Here's how the part is built. I have some questions about the finished solid (model axes, mm). Face numbers are marked on the shaded views. A direction names the side the tool comes from. Give positions to 0.01 mm unless a question says otherwise; leave off trailing zeros. Loops run counter-clockwise (first coordinate to the right, second up) from the corner with the lowest first, then second, coordinate; pieces in that order, holes last. Notation, with made-up numbers: (52, 26) - (66, 26) arc R29 ccw to (66, 65) - close; hole circle Ø4 at (56, -3.75). An arc over 180 degrees is marked (long way). Use a Markdown table: item, result.
from build123d import *

# Parameters (mm, degrees)
CYLINDER_R        = 1.45
CYLINDER_DEPTH    = 20
ARRAY_Y_COUNT     = 2
ARRAY_Y_PITCH     = 9
BOX002_W          = 5
BOX002_H          = 14.5
BOX002_DEPTH      = 2
BOX003_W          = 2
BOX003_H          = 14.5
BOX003_DEPTH      = 2
CYLINDER001_R     = 1.8
CYLINDER001_DEPTH = 10
ARRAY002_Y_COUNT  = 2
ARRAY002_Y_PITCH  = 30
BOX004_W          = 9.6
BOX004_H          = 40
BOX004_DEPTH      = 2
FILLET_R          = 4
BOX001_W          = 16
BOX001_H          = 14.5
BOX001_DEPTH      = 3.5
BOX_W             = 17
BOX_H             = 16.5
BOX_DEPTH         = 5.5


with BuildPart() as hole_array:
    # Cylinder → Cylinder (new body)
    with BuildSketch(Plane(origin=(7, 3.75, 0), x_dir=(1, 0, 0), z_dir=(0, 0, 1))):
        Circle(CYLINDER_R)
    extrude(amount=CYLINDER_DEPTH)

    # Array Y: hole array ×2


with BuildPart() as hole_array_1:
    add(hole_array.part)
    with Locations(*[(0, i * ARRAY_Y_PITCH, 0) for i in range(1, ARRAY_Y_COUNT)]):
        add(hole_array.part)


with BuildPart() as hole_stand_cube:
    # Box002 → Box002 (new body)
    with BuildSketch(Plane(origin=(4.5, 1, 2), x_dir=(1, 0, 0), z_dir=(0, 0, 1))):
        with Locations((2.5, 7.25)):
            Rectangle(BOX002_W, BOX002_H)
    extrude(amount=BOX002_DEPTH)


with BuildPart() as obj1:
    # Box003 → Box003 (new body)
    with BuildSketch(Plane(origin=(12, 1, 2), x_dir=(1, 0, 0), z_dir=(0, 0, 1))):
        with Locations((1, 7.25)):
            Rectangle(BOX003_W, BOX003_H)
    extrude(amount=BOX003_DEPTH)


with BuildPart() as attach_hole_array:
    # Cylinder001 → Cylinder001 (new body)
    with BuildSketch(Plane(origin=(4.8, 5, 0), x_dir=(1, 0, 0), z_dir=(0, 0, 1))):
        Circle(CYLINDER001_R)
    extrude(amount=CYLINDER001_DEPTH)

    # Array002 Y: attach hole array ×2


with BuildPart() as attach_hole_array_1:
    add(attach_hole_array.part)
    with Locations(*[(0, i * ARRAY002_Y_PITCH, 0) for i in range(1, ARRAY002_Y_COUNT)]):
        add(attach_hole_array.part)


with BuildPart() as attach_plane:
    # Box004 → Box004 (new body)
    with BuildSketch(Plane.XY):
        with Locations((4.8, 20)):
            Rectangle(BOX004_W, BOX004_H)
    extrude(amount=BOX004_DEPTH)

    # Fillet
    fillet_edges = [attach_plane.edges().sort_by_distance(p)[0] for p in [
        (0, 0, 1),
        (0, 40, 1),
        (9.6, 0, 1),
        (9.6, 40, 1),
    ]]
    fillet(fillet_edges, radius=FILLET_R)

    # Cut002: cut attach hole array
    add(attach_hole_array_1.part, mode=Mode.SUBTRACT)


with BuildPart() as attach_plane_1:
    # Cut002 placement: moved
    add(attach_plane.part.moved(Location((3.7, -11.75, 0))))


with BuildPart() as bottom_cube_extract:
    # Box001 → Box001 (new body)
    with BuildSketch(Plane(origin=(1, 1, 2), x_dir=(1, 0, 0), z_dir=(0, 0, 1))):
        with Locations((8, 7.25)):
            Rectangle(BOX001_W, BOX001_H)
    extrude(amount=BOX001_DEPTH)


with BuildPart() as obj2:
    # Box → Box (new body)
    with BuildSketch(Plane.XY):
        with Locations((8.5, 8.25)):
            Rectangle(BOX_W, BOX_H)
    extrude(amount=BOX_DEPTH)

    # Cut: cut bottom cube extract
    add(bottom_cube_extract.part, mode=Mode.SUBTRACT)

    # Fusion: union hole stand cube, obj1, attach plane
    add(hole_stand_cube.part)
    add(obj1.part)
    add(attach_plane_1.part)

    # Cut001: cut hole array
    add(hole_array_1.part, mode=Mode.SUBTRACT)


solid = obj2.part
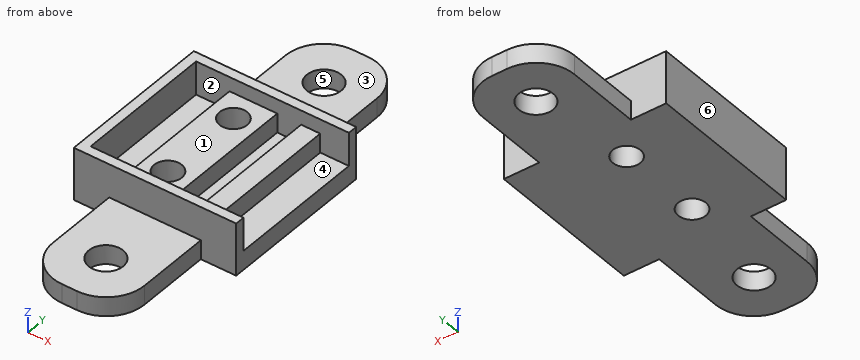
(1) Suppose I cut it at A-A on y = 12.75. Write out the boundary of the cut face in (x, z), plus the area to 3 significant figures.
A:
| item | result |
|---|---|
| outline | (0, 0) - (5.55, 0) - (5.55, 4) - (4.5, 4) - (4.5, 2) - (1, 2) - (1, 5.5) - (0, 5.5) - close; (8.45, 0) - (17, 0) - (17, 2) - (14, 2) - (14, 4) - (12, 4) - (12, 2) - (9.5, 2) - (9.5, 4) - (8.45, 4) - close |
| area | 39.9 mm2 |
(2) If I drill on line 1 (X direction, y = 6, z = 2.2); line 2 (Y direction, x = 8.5, z = 1); line 3 (X direction, y = -6.75, z = 1.2), over which ranges is the centre line in solid material (lowest first)?
A:
| item | result |
|---|---|
| line 1 | 0 to 1, 4.5 to 9.5, 12 to 14 |
| line 2 | -11.75 to -8.55, -4.95 to 21.45, 25.05 to 28.25 |
| line 3 | 3.7 to 6.7, 10.3 to 13.3 |
(3) Suppose I cut it at C-C on z = 4.6. Write out the boundary of the cut face in (x, y), plus the area to 3 significant figures.
A:
| item | result |
|---|---|
| outline | (0, 0) - (17, 0) - (17, 1) - (1, 1) - (1, 15.5) - (17, 15.5) - (17, 16.5) - (0, 16.5) - close |
| area | 48.5 mm2 |
(4) On a 3-axis mill with a long thin cutter (end or side, diameter ignored), from which of +Z, -Z, +X, -X, +Y, -Y can I reach the whole of each face in a straight line? I mean the marked faces 1, 2 and 3. Say none if no direction works.
A:
| item | result |
|---|---|
| face 1 | +Z, +X |
| face 2 | +Z |
| face 3 | +Z, +X, -X, +Y |
(5) Will these pins go through, and if not, where does the flat tip stop? pin 1 (2.5 mm diameter, centred on x = 15.5, y = 10.5, fed in from +Z); pin 2 (1.5 mm diameter, centred on x = 2, z = 1.5, fed in from -Y); pin 3 (3.5 mm diameter, centred on x = 7, y = 12.75, fed in from +Z).
A:
| item | result |
|---|---|
| pin 1 | z = 2 |
| pin 2 | y = 0 |
| pin 3 | z = 4 |
(6) We'd pull the mould along X, two halves only. Please class the marked faces 4, 5 and 6: pulls with the +X half, pulls with the -X half, needs draft (parallel to the pull), parting line crosses it, or undercut.
A:
| item | result |
|---|---|
| face 4 | needs draft |
| face 5 | undercut |
| face 6 | pulls with the -X half |
(7) Suppose I cut it at B-B on z = 2.7. Write out the boundary of the cut face in (x, y), plus the area to 3 significant figures.
A:
| item | result |
|---|---|
| outline | (0, 0) - (17, 0) - (17, 1) - (14, 1) - (14, 15.5) - (17, 15.5) - (17, 16.5) - (0, 16.5) - close; hole (1, 1) - (4.5, 1) - (4.5, 15.5) - (1, 15.5) - close; hole circle Ø2.9 at (7, 3.75); hole circle Ø2.9 at (7, 12.75); hole (9.5, 1) - (12, 1) - (12, 15.5) - (9.5, 15.5) - close |
| area | 137 mm2 |
(8) Suppose I cut it at D-D on y = 23.25. Write out the boundary of the cut face in (x, z), plus the area to 3 significant figures.
A:
| item | result |
|---|---|
| outline | (3.7, 0) - (6.7, 0) - (6.7, 2) - (3.7, 2) - close; (10.3, 0) - (13.3, 0) - (13.3, 2) - (10.3, 2) - close |
| area | 12.0 mm2 |
